from build123d import *

# Parameters (mm, degrees)
F1_DEPTH    = 4
F2_R        = 2
F0_W        = 10
F0_H        = 10
F3_DEPTH    = 11
F4_W        = 44.1
F4_H        = 10
F5_DEPTH    = 55
F6_T        = 1.5
F6_T3_DEPTH = 13
F6_T5_DEPTH = 47.1
F6_T7_DEPTH = 7
F6_T9_DEPTH = 27.1
F7_R        = 2


# Not quite as in the source:
# - a shell that OpenCascade refuses in one call is made with other operations: the cavity is built on its own and cut out


with BuildPart() as f1:
    # F0 (on Top) → F1 (new body)
    with BuildSketch(Plane.XY):
        Polygon((-12.05, 0), (0, 0), (12.05, 0), (12.05, 10), (-12.05, 10), align=None)
        Polygon((-12.05, 48.5), (-12.05, 10), (12.05, 10), (12.05, 48.5), (8.55, 45), (10.55, 45), (10.55, 23), (0, 23), (-10.55, 23), (-10.55, 45), (-8.55, 45), align=None)
    extrude(amount=F1_DEPTH)

    # F2
    f2_edges = [f1.edges().sort_by_distance(p)[0] for p in [
        (-10.55, 23, 2),
        (10.55, 23, 2),
    ]]
    fillet(f2_edges, radius=F2_R)

    # F0 (on Top) → F3 (join)
    with BuildSketch(Plane.XY):
        with Locations((17.05, 5)):
            Rectangle(F0_W, F0_H)
        Polygon((-12.05, 0), (0, 0), (12.05, 0), (12.05, 10), (-12.05, 10), align=None)
        with Locations((-17.05, 5)):
            Rectangle(F0_W, F0_H)
    extrude(amount=F3_DEPTH)

    # F4 (on face) → F5 (join)
    with BuildSketch(Plane.XY.offset(11)):
        Polygon((-27.5, 70), (-27.5, 0), (-22.05, 0), (-22.05, 10), (22.05, 10), (22.05, 0), (27.5, 0), (27.5, 70), align=None)
        with Locations((0, 5)):
            Rectangle(F4_W, F4_H)
    extrude(amount=F5_DEPTH)

    # F6: shell of thickness 1.5, made by hand


with BuildPart() as f6_core1:
    # F6_t2: copy of F1
    add(f1.part)

    # the walls: a layer under each face that stays
    f6_faces = [f6_core1.faces().sort_by_distance(p)[0] for p in [
        (-27.5, 35, 38.5),
        (0, 0, 33),
        (0, 35, 11),
        (0, 35, 66),
        (27.5, 35, 38.5),
        (22.05, 5, 5.5),
        (0, 10, 5.5),
        (-22.05, 5, 5.5),
        (-14.7, 8.0833333333, 0),
        (12.05, 29.25, 2),
        (-8.0333333333, 16.4166666667, 4),
        (-12.05, 29.25, 2),
        (10.55, 35, 2),
        (9.9642135624, 23.5857864376, 2),
        (0, 23, 2),
        (-9.9642135624, 23.5857864376, 2),
        (-10.55, 35, 2),
        (-9.55, 45, 2),
        (-10.3, 46.75, 2),
        (10.3, 46.75, 2),
        (9.55, 45, 2),
    ]]
    thicken(f6_faces, amount=-F6_T, mode=Mode.SUBTRACT)

    # F6_s4 → F6_t3 (cut)
    with BuildSketch(Plane.XZ.offset(-11.5)):
        Polygon((22.065, 10.985), (22.05, 12.5), (20.55, 12.5), (20.55, 11), align=None)
        Polygon((-22.065, 10.985), (-22.05, 12.5), (-20.55, 12.5), (-20.55, 11), align=None)
    extrude(amount=F6_T3_DEPTH, mode=Mode.SUBTRACT)

    # F6_s6 → F6_t5 (cut)
    with BuildSketch(Plane.YZ.offset(-23.55)):
        Polygon((10.015, 10.985), (10, 12.5), (8.5, 12.5), (8.5, 11), align=None)
    extrude(amount=F6_T5_DEPTH, mode=Mode.SUBTRACT)

    # F6_s8 → F6_t7 (cut)
    with BuildSketch(Plane.XY.offset(-1.5)):
        Polygon((12.065, 10.015), (12.05, 8.5), (10.55, 8.5), (10.55, 10), align=None)
        Polygon((-12.065, 10.015), (-12.05, 8.5), (-10.55, 8.5), (-10.55, 10), align=None)
        Polygon((10.535, 44.985), (12.05, 45), (12.05, 46.5), (10.55, 46.5), align=None)
        Polygon((-10.535, 44.985), (-12.05, 45), (-12.05, 46.5), (-10.55, 46.5), align=None)
    extrude(amount=F6_T7_DEPTH, mode=Mode.SUBTRACT)

    # F6_s10 → F6_t9 (cut)
    with BuildSketch(Plane.YZ.offset(-13.55)):
        Polygon((10.015, 4.015), (8.5, 4), (8.5, 2.5), (10, 2.5), align=None)
    extrude(amount=F6_T9_DEPTH, mode=Mode.SUBTRACT)


with BuildPart() as f1_1:
    add(f1.part)

    # what is left inside the walls is the cavity
    f6_cavity = [f6_core1.part.solids().sort_by_distance(p)[0] for p in [
        (-25.985, 35.75, 47.166667),
    ]]
    add(f6_cavity, mode=Mode.SUBTRACT)

    # F7
    f7_edges = [f1_1.edges().sort_by_distance(p)[0] for p in [
        (-27.5, 35, 66),
        (-27.5, 35, 11),
        (27.5, 35, 11),
        (27.5, 35, 66),
    ]]
    fillet(f7_edges, radius=F7_R)


solid = f1_1.part
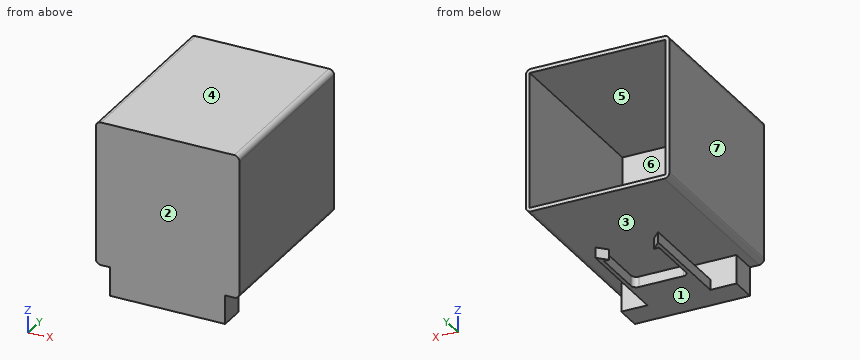
Design review of the part built by this model. Coordinates are the model's own, in mm. Face numbers are marked on the shaded views. A direction names the side the tool comes from. Round coordinates to 2 decimals unless told otherwise and drop trailing zeros. Write each loop counter-clockwise with the first axis right and the second up, starting at its lowest first coordinate (ties: lowest second). Pieces come first, ordered by that corner, then holes. Notation, with made-up numbers: (-8.5, 26.5) -> (0.5, 26.5) arc R24 cw to (0.5, 65.5) -> close; hole circle Ø4 at (-21, 70). An arc over 180 degrees is marked (long way). One line per item, written item: value. Start each with the question number.
Q1. Tool access review of the marked faces 5, 6 and 7: name each direction out of +Z, -Z, +X, -X, +Y, -Y from which nothing blocks a thin tool from reaching the whole face with its end or side.
Q2. Add section D-D (x = -14.5). Give the boundary of the cut face in (y, z).
Q3. Add section A-A (y = 28.5). Give the boundary of the cut face in (x, z), then the cut area to 3 significant figures.
Q4. To check wall thickness, follow probe 1 along Z at (x, y) = (12, 35); probe 2 along Y at (x, z) = (8, 8.5); probe 3 along X at (y, z) = (31.5, 63.5). State the ranges of each line that lie inside material, in increasing order.
Q5. The part is to be moulded in two halves that separate along Z. For the marked faces 1, 2, 3 and 4, say which applies: pulls with the +Z half, pulls with the -Z half, needs draft (parallel to the pull), parting line crosses it, or undercut.
Q6. Add section B-B (z = 7.5). Give the boundary of the cut face in (x, y).
Q7. Insertion check: P1, Ø2, axis at x = -9, z = 2.5, coming from the -Y side; P2, Ø3, axis at x = -13, z = 52, coming from the +Y side; P3, Ø5, axis at y = 5.5, z = 3, coming from the -X side; P4, Ø5.5, axis at y = 6.5, z = 4.5, coming from the +X side. Each pin has a flat end and moves straight along its axis. Give the tip position at first contact, or say it passes through.
Q8. Add section C-C (y = 60.5). Give the boundary of the cut face in (x, z).
Response:
1. face 5: +Y
1. face 6: none
1. face 7: +Z, -Z, -X, +Y, -Y
2. outline: (0, 0) -> (10, 0) -> (10, 11) -> (70, 11) -> (70, 12.5) -> (8.5, 12.5) -> (8.5, 1.5) -> (1.5, 1.5) -> (1.5, 64.5) -> (70, 64.5) -> (70, 66) -> (0, 66) -> close
3. outline: (-27.5, 13) arc R2 ccw to (-25.5, 11) -> (25.5, 11) arc R2 ccw to (27.5, 13) -> (27.5, 64) arc R2 ccw to (25.5, 66) -> (-25.5, 66) arc R2 ccw to (-27.5, 64) -> close; (-12.05, 0) -> (-10.55, 0) -> (-10.55, 4) -> (-12.05, 4) -> close; (10.55, 0) -> (12.05, 0) -> (12.05, 4) -> (10.55, 4) -> close; hole (-26, 12.5) -> (26, 12.5) -> (26, 64.5) -> (-26, 64.5) -> close
3. area: 330 mm^2
4. probe 1: z = 0 to 4, 11 to 12.5, 64.5 to 66
4. probe 2: y = 0 to 1.5, 8.5 to 10
4. probe 3: x = -27.5 to -26, 26 to 27.5
5. face 1: pulls with the -Z half
5. face 2: needs draft
5. face 3: undercut
5. face 4: pulls with the +Z half
6. outline: (-22.05, 0) -> (22.05, 0) -> (22.05, 10) -> (-22.05, 10) -> close; hole (-20.55, 1.5) -> (20.55, 1.5) -> (20.55, 8.5) -> (-20.55, 8.5) -> close
7. P1: stops at y = 0
7. P2: stops at y = 1.5
7. P3: stops at x = -22.05
7. P4: stops at x = 22.05
8. outline: (-27.5, 13) arc R2 ccw to (-25.5, 11) -> (25.5, 11) arc R2 ccw to (27.5, 13) -> (27.5, 64) arc R2 ccw to (25.5, 66) -> (-25.5, 66) arc R2 ccw to (-27.5, 64) -> close; hole (-26, 12.5) -> (26, 12.5) -> (26, 64.5) -> (-26, 64.5) -> close
